Autodesk Inventor part; units mm, degrees
ref_plane "YZ Plane" through (0, 0, 0) normal (1, 0, 0) x (0, 1, 0)
ref_plane "XZ Plane" through (0, 0, 0) normal (0, 1, 0) x (-1, 0, 0)
ref_plane "XY Plane" through (0, 0, 0) normal (0, 0, 1) x (1, 0, 0)
ref_plane "Plano de trabajo1" through (-15, 0, -15) normal (0, -1, 0) x (1, 0, 0)
sketch "Boceto2" plane through (-15, 0, -15) normal (0, -1, 0) x (1, 0, 0)
  line L0 (566, 15) -> (1911, 15)
  line L1 (566, 536) -> (566, 15)
  line L2 (1911, 536) -> (566, 536)
  line L3 (1911, 15) -> (1911, 536)
  line L4 (536, 1414) -> (15, 1414)
  line L5 (536, 15) -> (536, 1414)
  line L6 (15, 15) -> (536, 15)
  line L7 (15, 1414) -> (15, 15)
  line L8 (-15, 1444) -> (566, 1444)
  line L9 (-15, -15) -> (-15, 1444)
  line L10 (1941, -15) -> (-15, -15)
  line L11 (1941, 566) -> (1941, -15)
  line L12 (566, 566) -> (1941, 566)
  line L13 (566, 1444) -> (566, 566)
  line L14 (566, 566) -> (566, 544.7868)
  line L15 (6.2132, -15) -> (15, -15)
  line L16 (544.7868, 566) -> (-15, 6.2132)
  line L17 (566, 544.7868) -> (6.2132, -15)
  line L18 (566, 566) -> (544.7868, 566)
  line L19 (-15, 6.2132) -> (-15, -15)
  line L20 (6.2132, -15) -> (-15, -15)
  point P0 (6.2132, -15)
  dimension "d4" = 30
  dimension "d6" = 30
extrude "Extrusión2" add sketch "Boceto2" against normal blind 770 contours L16 L18 L14 L17 L5 | L5 L17 L6 L7 L16 | L7 L6 L17 L10 L9 L16
sketch "Boceto3" plane through (-15, 0, -15) normal (0, -1, 0) x (1, 0, 0)
  line L0 (566, 544.7868) -> (566, 566)
  line L1 (566, 566) -> (544.7868, 566)
  line L2 (544.7868, 566) -> (-15, 6.2132)
  line L3 (-15, 6.2132) -> (-15, -15)
  line L4 (-15, -15) -> (6.2132, -15)
  line L5 (6.2132, -15) -> (566, 544.7868)
  line L6 (-15, -15) -> (15, -15)
  line L7 (15, -15) -> (15, 15)
  line L8 (15, 15) -> (-15, 15)
  line L9 (-15, 15) -> (-15, -15)
  point P0 (-6.2132, 15)
  point P1 (15, -6.2132)
  dimension "d9" = 30
  dimension "d10" = 30
extrude "Extrusión3" cut sketch "Boceto3" against normal blind 770 contours L5 L4 L3 L2 L8 L7
sketch "Boceto4" plane through (551, 0, 529.7868) normal (0.7071, 0, -0.7071) x (-0.7071, 0, -0.7071)
  line L0 (764.2317, 0) -> (764.2317, 770)
  line L1 (764.2317, 0) -> (764.2317, 770)
  line L2 (779.2317, 0) -> (764.2317, 0)
  line L3 (-9.9264, 770) -> (764.2317, 0)
  line L4 (13.656, 788.8569) -> (806.7728, 0)
  line L5 (779.2317, 0) -> (779.2317, 770)
  line L6 (0, 770) -> (779.2317, 770)
  line L7 (0, 0) -> (0, 770)
  line L8 (779.2317, 0) -> (0, 0)
  line L9 (0, 0) -> (-15, 0)
  line L10 (0, 0) -> (0, 770)
  line L11 (-15, 770) -> (0, 770)
  line L12 (-15, 0) -> (-15, 770)
  line L13 (779.2317, 0) -> (779.2317, 770)
  line L14 (0, 770) -> (779.2317, 770)
  line L15 (0, 0) -> (0, 770)
  line L16 (779.2317, 0) -> (0, 0)
  point P0 (32.6148, 770)
  point P1 (779.2317, 27.3932)
  point P2 (764.2317, 0)
  dimension "d13" = 30
extrude "Extrusión4" cut sketch "Boceto4" against normal blind 770 contours L8 L7 L3 | L4 L6 L0 | L0 L6 L5 L4 | L7 L9 L12 L11 L3
properties part number "Barra inversa"
Read the model definition and answer for the solid it produces. Units are mm, in the model's axes. A direction names the side the tool comes from. Coordinates: 2 decimals unless noted, no trailing zeros. Loops run counter-clockwise (first coordinate to the right, second up) from the corner with the lowest first, then second, coordinate; pieces in that order, holes last. Notation, with made-up numbers: (34, -6) -> (55, -6) arc R26 cw to (55, 18) -> close; hole circle Ø1 at (53.25, 45.5). An arc over 180 degrees is marked (long way). Return JSON: item names as keys, results as strings.
Item 1: Find section A-A (z = 326.5). Determine the outline of the cut face in (x, y).
Answers:
{"outline": "(305.29, 444.34) -> (347.71, 474.18) -> (347.71, 516.49) -> (305.29, 486.65) -> close"}
Item 2: Flat-ended cylindrical pins translate along their axes: P1, Ø5, axis at y = 336.5, z = 234, coming from the +X side; P2, Ø6, axis at y = 206, z = 103, coming from the -X side; P3, Ø12, axis at x = 61.5, y = 104.5, coming from the -Z side. Find the tip coordinate at first contact, or state that the pin passes through.
Answers:
{"P1": "stops at x = 248.8", "P2": "stops at x = 124.52", "P3": "stops at z = 34.29"}
Item 3: Find section B-B (x = 295.5). Determine the outline of the cut face in (y, z).
Answers:
{"outline": "(400.74, 274.29) -> (443.05, 274.29) -> (472.89, 316.71) -> (430.57, 316.71) -> close"}
Item 4: For faces 1 (the flat face through (277.69, 390.39, 277.39)), 2 (the flat face through (-10, 16, 0)), determine the directions among +Z, -Z, +X, -X, +Y, -Y from which every point of the face is accessible in a straight line to the end or side of a thin tool.
Answers:
{"face 1": "+Z, +X, -Y", "face 2": "-Z, -X, +Y, -Y"}
Item 5: Find the intervals of material crossed by probe 1 along Z at (x, y) = (457, 645); probe 2 along Z at (x, y) = (453, 653.5), in increasing order.
Answers:
{"probe 1": "z = 435.79 to 460.09", "probe 2": "z = 431.79 to 474.21"}
